The model under review builds one solid part; all positions refer to its coordinate system, in mm. Face numbers are marked on the shaded views. Round coordinates to 2 decimals unless told otherwise and drop trailing zeros. Write each loop counter-clockwise with the first axis right and the second up, starting at its lowest first coordinate (ties: lowest second). Pieces come first, ordered by that corner, then holes. Notation, with made-up numbers: (81.5, 23) -> (138.5, 23) arc R23 cw to (138.5, 34) -> close; hole circle Ø4 at (0.25, 80). An arc over 180 degrees is marked (long way). Answer as a JSON object with one key per item and string values. Group by question number.
1) Insertion check: pin 1 Ø6 at (x, y) = (-8.5, 230.5) entering from +Z; pin 2 Ø2.5 at (y, z) = (237, 18) entering from -X; pin 3 Ø1 at (x, y) = (-75.5, -152.5) entering from -Z; pin 4 Ø6.5 at (y, z) = (-236.5, 17) entering from +X. Each pin has a flat end and moves straight along its axis. Give the tip position at first contact, or say it passes through.
2) We need section B-B, the plane x = 56.5. Write out the cut boundary in (y, z), then the cut area to 3 significant figures.
3) Mouldability with a two-part tool opening along X and no side actions: class the marked faces 1 and 2 as pulls with the +X half, pulls with the -X half, needs draft (parallel to the pull), parting line crosses it, or undercut.
4) To check wall thickness, follow probe 1 along Y at (x, z) = (92.5, 12.75); probe 2 along X at (y, z) = (15, 20); probe 3 along Z at (x, y) = (-63, -98). State the ranges of each line that lie inside material, in increasing order. Write a range as [from, to].
5) We need section A-A, the plane y = -35. Write out the cut boundary in (x, z), then the cut area to 3 significant figures.
from build123d import *

# Parameters (mm, degrees)
F1_DEPTH = 22
F3_DEPTH = 18
F4_R     = 8
F5_W     = 30
F5_H     = 597.1070975065
F6_DEPTH = 8
F7_R     = 5


with BuildPart() as f1:
    # F0 (on Top) → F1 (new body)
    with BuildSketch(Plane.XY):
        with BuildLine():
            Line((200, 245), (0, 245))
            Line((0, 245), (-200, 245))
            ThreePointArc((-200, 245), (-214.1421356237, 239.1421356237), (-220, 225))
            Line((-220, 225), (-220, 0))
            Line((-220, 0), (-220, -225))
            ThreePointArc((-220, -225), (-214.1421356237, -239.1421356237), (-200, -245))
            Line((-200, -245), (0, -245))
            Line((0, -245), (200, -245))
            ThreePointArc((200, -245), (214.1421356237, -239.1421356237), (220, -225))
            Line((220, -225), (220, 0))
            Line((220, 0), (220, 225))
            ThreePointArc((220, 225), (214.1421356237, 239.1421356237), (200, 245))
        make_face()
    extrude(amount=F1_DEPTH)

    # F2 (on face) → F3 (cut)
    with BuildSketch(Plane.XY.offset(22)):
        with BuildLine():
            Line((190, 225), (-190, 225))
            ThreePointArc((-190, 225), (-197.0710678119, 222.0710678119), (-200, 215))
            Line((-200, 215), (-200, -215))
            ThreePointArc((-200, -215), (-197.0710678119, -222.0710678119), (-190, -225))
            Line((-190, -225), (190, -225))
            ThreePointArc((190, -225), (197.0710678119, -222.0710678119), (200, -215))
            Line((200, -215), (200, 215))
            ThreePointArc((200, 215), (197.0710678119, 222.0710678119), (190, 225))
        make_face()
    extrude(amount=-F3_DEPTH, mode=Mode.SUBTRACT)

    # F4
    f4_edges = [f1.edges().sort_by_distance(p)[0] for p in [
        (0, 225, 4),
        (-197.071068, 222.071068, 4),
        (-200, 0, 4),
        (-197.071068, -222.071068, 4),
        (0, -225, 4),
        (197.071068, -222.071068, 4),
        (200, 0, 4),
        (197.071068, 222.071068, 4),
    ]]
    fillet(f4_edges, radius=F4_R)

    # F5 (on face) → F6 (cut)
    with BuildSketch(Plane.XY.offset(22)):
        with Locations((0, -8.4120258689)):
            Rectangle(F5_W, F5_H)
    extrude(amount=-F6_DEPTH, mode=Mode.SUBTRACT)

    # F7
    f7_edges = [f1.edges().sort_by_distance(p)[0] for p in [
        (-15, -245, 18),
        (15, -245, 18),
        (15, -225, 18),
        (-15, -225, 18),
        (-15, 225, 18),
        (-15, 245, 18),
        (15, 225, 18),
        (15, 245, 18),
    ]]
    fillet(f7_edges, radius=F7_R)


solid = f1.part
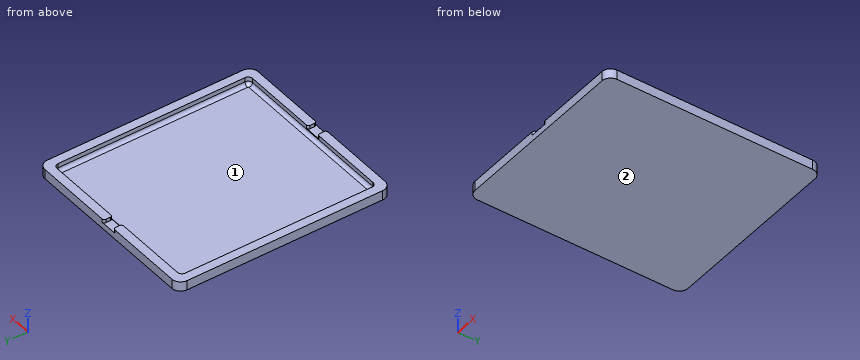
Here are the results:
{
 "1": {"pin 1": "stops at z = 14", "pin 2": "stops at x = -216.87", "pin 3": "stops at z = 0", "pin 4": "stops at x = 218.22"},
 "2": {"outline": "(-245, 0) -> (245, 0) -> (245, 22) -> (225, 22) -> (225, 12) arc R8 cw to (217, 4) -> (-217, 4) arc R8 cw to (-225, 12) -> (-225, 22) -> (-245, 22) -> close", "area": "2,710 mm^2"},
 "3": {"face 1": "undercut", "face 2": "needs draft"},
 "4": {"probe 1": "y = [-245, -225], [225, 245]", "probe 2": "x = [-220, -200], [200, 220]", "probe 3": "z = [0, 4]"},
 "5": {"outline": "(-220, 0) -> (220, 0) -> (220, 22) -> (200, 22) -> (200, 12) arc R8 cw to (192, 4) -> (-192, 4) arc R8 cw to (-200, 12) -> (-200, 22) -> (-220, 22) -> close", "area": "2,510 mm^2"}
}
